The listing builds one solid part. Answer for the finished solid, in the listing's coordinates (mm). A direction names the side the tool comes from. Coordinates: 2 decimals unless noted, no trailing zeros. Order: outer loops, then holes, each group sorted by start corner. A loop starts at its lowest first (then second) coordinate and runs counter-clockwise, first axis right, second up. Notation, with made-up numbers: (-1, 2) - (54, 2) arc R23 ccw to (54, 32) - close; hole circle Ø10 at (-8, 17.25). An arc over 180 degrees is marked (long way). Use one line per item in the form item = value. Start each with the question number.
Item 1: Each of these flat-tipped pins is pushed along its axis until it touches: pin 1 Ø1 at (y, z) = (0, 9) entering from -X; pin 2 Ø1.5 at (x, y) = (-16.5, 0.5) entering from +Z; pin 3 Ø2.5 at (y, z) = (0.5, 37) entering from +X. Where does it stop, or does it pass through?
Item 2: Section B-B, the plane z = 23 is taken. Write down the section's boundary in (x, y), and give its area (3 significant figures).
Item 3: Section A-A, the plane x = -37.5 is taken. Write down the section's boundary in (y, z), and give its area (3 significant figures).
Item 4: Consider line 1 along X through (y, z) = (-0.55, 38); line 2 along X through (y, z) = (1.8, 0); line 3 along Z through (x, y) = (-11, -0.5). Determine where each line is inside the solid, lowest interval first. Write a range as [from, to].
Item 5: A tool of negligible diameter and unlimited length cuts with its end or side. For faces 5 (the flat face through (-35, -2.5, 7)), 6 (the flat face through (-9.683, 0, 37)), from which of +Z, -Z, +X, -X, +Y, -Y can it reach the whole face along a straight path? Write none if from no direction.
Item 6: The mould has two halves that part along X. Classify faces 1 (the cylindrical face through (-29.2, 0, 33.9)), 2 (the flat face through (-37, 0, 42.637)), 3 (the flat face through (-45.467, 0, 29)), 4 (the cylindrical face through (-27.947, 0.035, 17.549)): released by +X, released by -X, zero draft, split by the parting line, or undercut.
from build123d import *

# Parameters (mm, degrees)
BOSS_EXTRUDE1_DEPTH = 2.5
SKETCH2_W           = 39
SKETCH2_H           = 19
CUT_EXTRUDE2_DEPTH  = 119.291735722
SKETCH6_R           = 1.5
CUT_EXTRUDE11_DEPTH = 119.291735722
CUT_EXTRUDE17_DEPTH = 10
SKETCH17_W          = 77.591598172
SKETCH17_H          = 70.367911795
CUT_EXTRUDE19_DEPTH = 10
CUT_EXTRUDE20_DEPTH = 10
SKETCH18_W          = 37.449354942
SKETCH18_H          = 14.815690613
CUT_EXTRUDE21_DEPTH = 10


with BuildPart() as part:
    # Sketch1 → Boss-Extrude1 (new, symmetric)
    with BuildSketch(Plane(origin=(0, 0, 0), x_dir=(1, 0, 0), z_dir=(0, 1, 0))):
        with BuildLine():
            Line((25.786244138, -33), (0, -33))
            ThreePointArc((0, -33), (-33, 0), (0, 33))
            Line((0, 33), (0, 48))
            ThreePointArc((0, 48), (-39.003855832, 27.976762325), (-45.466733516, -15.387532074))
            Line((-45.466733516, -15.387532074), (-45.466733516, -107.999697871))
            Line((-45.466733516, -107.999697871), (25.786244138, -107.999697871))
            Line((25.786244138, -107.999697871), (25.786244138, -33))
        make_face()
        with BuildLine():
            Line((-7.096269411, -47.472549547), (0, -47.472549547))
            Line((0, -47.472549547), (0, -48))
            ThreePointArc((0, -48), (-3.55792227, -47.867955765), (-7.096269411, -47.472549547))
        make_face(mode=Mode.SUBTRACT)
    extrude(amount=BOSS_EXTRUDE1_DEPTH, both=True)

    # Sketch2 → Cut-Extrude2 (cut, through all)
    with BuildSketch(Plane(origin=(0, 2.5, 0), x_dir=(1, 0, 0), z_dir=(0, 1, 0))):
        with Locations((-9.786245396, -52.095481266)):
            Rectangle(SKETCH2_W, SKETCH2_H)
    extrude(amount=-CUT_EXTRUDE2_DEPTH, mode=Mode.SUBTRACT)

    # Sketch6 → Cut-Extrude11 (cut, through all)
    with BuildSketch(Plane(origin=(0, 2.5, 0), x_dir=(1, 0, 0), z_dir=(0, 1, 0))):
        with Locations(Location((-30.466733516, -33.095481266, 0), (0, 0, 270))):
            Circle(SKETCH6_R)
    extrude(amount=-CUT_EXTRUDE11_DEPTH, mode=Mode.SUBTRACT)

    # Sketch11 → Cut-Extrude17 (cut)
    with BuildSketch(Plane(origin=(0, 2.5, 0), x_dir=(1, 0, 0), z_dir=(0, 1, 0))):
        with BuildLine():
            Line((-8.49120153, 39.220810677), (-8.49120153, 31.888861638))
            Line((-8.49120153, 31.888861638), (-32.514043682, 5.642425314))
            add(Edge.make_bspline(
                [(-32.514043682, 5.642425314), (-33.882768602, 31.207106787), (-8.49120153, 39.220810677)],
                knots=[0, 0, 0, 1, 1, 1], degree=2))
        make_face()
    extrude(amount=-CUT_EXTRUDE17_DEPTH, mode=Mode.SUBTRACT)

    # Sketch17 → Cut-Extrude19 (cut)
    with BuildSketch(Plane(origin=(0, 2.5, 0), x_dir=(1, 0, 0), z_dir=(0, 1, 0))):
        with Locations((-13.009554948, -77.820837223)):
            Rectangle(SKETCH17_W, SKETCH17_H)
    extrude(amount=-CUT_EXTRUDE19_DEPTH, mode=Mode.SUBTRACT)

    # Sketch16 → Cut-Extrude20 (cut)
    with BuildSketch(Plane(origin=(0, 2.5, 0), x_dir=(1, 0, 0), z_dir=(0, 1, 0))):
        with BuildLine():
            Line((0, 33), (0, 44.891139614))
            add(Edge.make_bspline(
                [(-8.49120153, 39.220810677), (-0.101410447, 43.066470158), (0, 44.891139614)],
                knots=[0, 0, 0, 0.444669129, 0.444669129, 0.444669129], degree=2))
            Line((-8.49120153, 39.220810677), (-8.49120153, 31.888861638))
            ThreePointArc((-8.49120153, 31.888861638), (-4.281796699, 32.721036307), (0, 33))
        make_face()
        with BuildLine():
            ThreePointArc((0, 48), (-6.393855284, 47.572246264), (-12.673752424, 46.296608942))
            add(Edge.make_bspline(
                [(0, 44.979230614), (-0.124166201, 47.152790476), (-12.673752424, 46.296608942)],
                knots=[0.455550409, 0.455550409, 0.455550409, 1, 1, 1], degree=2))
            Line((0, 44.979230614), (0, 48))
        make_face()
    extrude(amount=-CUT_EXTRUDE20_DEPTH, mode=Mode.SUBTRACT)

    # Sketch18 → Cut-Extrude21 (cut)
    with BuildSketch(Plane(origin=(0, 2.5, 0), x_dir=(1, 0, 0), z_dir=(0, 1, 0))):
        with Locations((9.041844157, -37.897729007)):
            Rectangle(SKETCH18_W, SKETCH18_H)
    extrude(amount=-CUT_EXTRUDE21_DEPTH, mode=Mode.SUBTRACT)


solid = part.part
Response:
q1.pin_1 = -47.24
q1.pin_2 = 42.6
q1.pin_3 = -9.68
q2.outline = (-45.47, -2.5) - (-23.66, -2.5) - (-23.66, 2.5) - (-45.47, 2.5) - close
q2.area = 109 mm2
q3.outline = (-2.5, -29.96) - (2.5, -29.96) - (2.5, 42.64) - (-2.5, 42.64) - close
q3.area = 363 mm2
q4.line_1 = [-45.47, -9.68]
q4.line_2 = [-48, -33]
q4.line_3 = [-46.4, -38.36], [31.11, 42.6]
q5.face_5 = +Z, -Z, +X, -X, -Y
q5.face_6 = +Z, +X, +Y, -Y
q6.face_1 = undercut
q6.face_2 = zero draft
q6.face_3 = released by -X
q6.face_4 = released by +X
